Part model, mm, in its own coordinate system. Face numbers are marked on the shaded views. A direction names the side the tool comes from. Round coordinates to 2 decimals unless told otherwise and drop trailing zeros. Loops run counter-clockwise (first coordinate to the right, second up) from the corner with the lowest first, then second, coordinate; pieces in that order, holes last. Notation, with made-up numbers: M 28,-5 L 37,-5 A13 ccw 37,11 Z; hole C 21,73.25 d9. An arc over 180 degrees is marked long. Put each result on its own line as item: value. Start each with the question number.
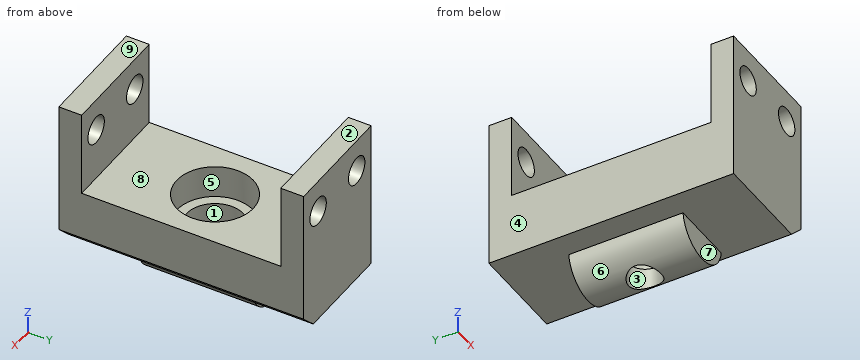
```python
from build123d import *

# Parameters (mm, degrees)
CYLINDER036_R          = 3.5
CYLINDER036_DEPTH      = 30
CYLINDER035_R          = 4.7
CYLINDER035_DEPTH      = 30
CYLINDER065_R          = 2
CYLINDER065_DEPTH      = 62
CYLINDER066_R          = 4
CYLINDER066_DEPTH      = 14
CYLINDER066_ROLL_ANGLE = 90
CYLINDER030_R          = 1.7
CYLINDER030_DEPTH      = 19
CYLINDER030_ROLL_ANGLE = 90
CYLINDER033_R          = 1.7
CYLINDER033_DEPTH      = 19
CYLINDER033_ROLL_ANGLE = 90
CYLINDER034_R          = 1.7
CYLINDER034_DEPTH      = 19
CYLINDER034_ROLL_ANGLE = 90
CYLINDER029_R          = 1.7
CYLINDER029_DEPTH      = 19
CYLINDER029_ROLL_ANGLE = 90
BOX001012_W            = 14
BOX001012_H            = 2.8
BOX001012_DEPTH        = 11
BOX001011_W            = 14
BOX001011_H            = 2.8
BOX001011_DEPTH        = 11
BOX001010_W            = 14
BOX001010_H            = 30
BOX001010_DEPTH        = 8
CHAMFER011_SIZE        = 2


with BuildPart() as cylinder036:
    # Cylinder036 → Cylinder036 (new body)
    with BuildSketch(Plane.XY.offset(-9)):
        Circle(CYLINDER036_R)
    extrude(amount=CYLINDER036_DEPTH)


with BuildPart() as bearing_nut:
    # Cylinder035 → Cylinder035 (new body)
    with BuildSketch(Plane.XY.offset(-4.5)):
        Circle(CYLINDER035_R)
    extrude(amount=CYLINDER035_DEPTH)

    # Fusion080: union Cylinder036
    add(cylinder036.part)


with BuildPart() as cylinder065:
    # Cylinder065 → Cylinder065 (new body)
    with BuildSketch(Plane.XY.offset(-59)):
        Circle(CYLINDER065_R)
    extrude(amount=CYLINDER065_DEPTH)


with BuildPart() as cut035:
    # Cylinder066 → Cylinder066 (new body)
    with BuildSketch(Plane.XY):
        Circle(CYLINDER066_R)
    extrude(amount=CYLINDER066_DEPTH)


with BuildPart() as cut035_1:
    # Cylinder066 roll: moved
    add(cut035.part.rotate(Axis((0, 0, 0), (1, 0, 0)), CYLINDER066_ROLL_ANGLE))


with BuildPart() as cut035_2:
    # Cylinder066 placement: moved
    add(cut035_1.part.moved(Location((0, 7, -8))))

    # Cut035: cut Cylinder065
    add(cylinder065.part, mode=Mode.SUBTRACT)


with BuildPart() as cylinder030:
    # Cylinder030 → Cylinder030 (new body)
    with BuildSketch(Plane.XY):
        Circle(CYLINDER030_R)
    extrude(amount=CYLINDER030_DEPTH)


with BuildPart() as cylinder030_1:
    # Cylinder030 roll: moved
    add(cylinder030.part.rotate(Axis((0, 0, 0), (1, 0, 0)), CYLINDER030_ROLL_ANGLE))


with BuildPart() as cylinder030_2:
    # Cylinder030 placement: moved
    add(cylinder030_1.part.moved(Location((4, 24, 6))))


with BuildPart() as cylinder033:
    # Cylinder033 → Cylinder033 (new body)
    with BuildSketch(Plane.XY):
        Circle(CYLINDER033_R)
    extrude(amount=CYLINDER033_DEPTH)


with BuildPart() as cylinder033_1:
    # Cylinder033 roll: moved
    add(cylinder033.part.rotate(Axis((0, 0, 0), (1, 0, 0)), CYLINDER033_ROLL_ANGLE))


with BuildPart() as cylinder033_2:
    # Cylinder033 placement: moved
    add(cylinder033_1.part.moved(Location((4, 24, 6))))


with BuildPart() as part_mirroring002:
    # Part__Mirroring002: instance of Cylinder033
    add(cylinder033_2.part.mirror(Plane(origin=(0, 0, 0), x_dir=(1, 0, 0), z_dir=(0, 1, 0))))


with BuildPart() as cylinder034:
    # Cylinder034 → Cylinder034 (new body)
    with BuildSketch(Plane.XY):
        Circle(CYLINDER034_R)
    extrude(amount=CYLINDER034_DEPTH)


with BuildPart() as cylinder034_1:
    # Cylinder034 roll: moved
    add(cylinder034.part.rotate(Axis((0, 0, 0), (1, 0, 0)), CYLINDER034_ROLL_ANGLE))


with BuildPart() as cylinder034_2:
    # Cylinder034 placement: moved
    add(cylinder034_1.part.moved(Location((-4, 24, 6))))


with BuildPart() as part_mirroring003:
    # Part__Mirroring003: instance of Cylinder034
    add(cylinder034_2.part.mirror(Plane(origin=(0, 0, 0), x_dir=(1, 0, 0), z_dir=(0, 1, 0))))


with BuildPart() as m3_clear_a:
    # Cylinder029 → Cylinder029 (new body)
    with BuildSketch(Plane.XY):
        Circle(CYLINDER029_R)
    extrude(amount=CYLINDER029_DEPTH)


with BuildPart() as m3_clear_a_1:
    # Cylinder029 roll: moved
    add(m3_clear_a.part.rotate(Axis((0, 0, 0), (1, 0, 0)), CYLINDER029_ROLL_ANGLE))


with BuildPart() as m3_clear_a_2:
    # Cylinder029 placement: moved
    add(m3_clear_a_1.part.moved(Location((-4, 24, 6))))

    # Fusion057: union Cylinder030, Part__Mirroring002, Part__Mirroring003
    add(cylinder030_2.part)
    add(part_mirroring002.part)
    add(part_mirroring003.part)


with BuildPart() as cube010:
    # Box001012 → Box001012 (new body)
    with BuildSketch(Plane(origin=(-7, 12.2, -1), x_dir=(1, 0, 0), z_dir=(0, 0, 1))):
        with Locations((7, 1.4)):
            Rectangle(BOX001012_W, BOX001012_H)
    extrude(amount=BOX001012_DEPTH)


with BuildPart() as cube009:
    # Box001011 → Box001011 (new body)
    with BuildSketch(Plane(origin=(-7, -15, -1), x_dir=(1, 0, 0), z_dir=(0, 0, 1))):
        with Locations((7, 1.4)):
            Rectangle(BOX001011_W, BOX001011_H)
    extrude(amount=BOX001011_DEPTH)


with BuildPart() as bearing_clamp:
    # Box001010 → Box001010 (new body)
    with BuildSketch(Plane(origin=(-7, -15, -8.5), x_dir=(1, 0, 0), z_dir=(0, 0, 1))):
        with Locations((7, 15)):
            Rectangle(BOX001010_W, BOX001010_H)
    extrude(amount=BOX001010_DEPTH)

    # Fusion055: union Cube010, Cube009
    add(cube010.part)
    add(cube009.part)

    # Cut006: cut M3-clear-a
    add(m3_clear_a_2.part, mode=Mode.SUBTRACT)

    # Fusion081: union Cut035
    add(cut035_2.part)

    # Cut036: cut bearing-nut
    add(bearing_nut.part, mode=Mode.SUBTRACT)

    # Chamfer011
    chamfer011_edges = [bearing_clamp.edges().sort_by_distance(p)[0] for p in [
        (7, 0, -8.5),
    ]]
    chamfer(chamfer011_edges, length=CHAMFER011_SIZE)


solid = bearing_clamp.part
```
1. Cut at B-B, the plane x = 0. Give the cut face in (y, z), and give its area (3 significant figures).
2. Wall check: L1, parallel to Z at x = 4, y = -12.75; L2, parallel to Y at x = -1, z = -0.25; L3, parallel to Y at x = 0, z = -11.2. Give the ranges that are in metal, low to high.
3. Cut at C-C, the plane y = -0.5. Give the cut face in (x, z), and give its area (3 significant figures).
4. Cut at A-A, the plane z = 1.5. Give the cut face in (x, y), and give its area (3 significant figures).
5. Mould opens along X. For the marked faces 1, 2, 3 and 4 say: released by +X, released by -X, zero draft, split by the parting line, or undercut.
6. Drop flat-ended pins along their axis: pin 1 (2.5 mm diameter, centred on x = -4, z = 6, fed in from +Y); pin 2 (5 mm diameter, centred on x = 1, y = -5.5, fed in from +Z); pin 3 (3 mm diameter, centred on x = -1, z = -11, fed in from +Y); pin 4 (6 mm diameter, centred on x = -3.5, y = 7, fed in from -Z). Give the stop position or say it passes through.
7. Cut at D-D, the plane z = 6. Give the cut face in (x, y), and give its area (3 significant figures).
8. Which spindle directions (+Z, -Z, +X, -X, +Y, -Y) get a long thin tool onto all of the face, cutting with end or side? Do the marked faces 5, 6, 7, 8 and 9. Say none if no direction does.
Results list:
1. outline: M -15,-8.5 L -7,-8.5 L -7,-12 L -2,-12 L -2,-9 L -3.5,-9 L -3.5,-4.5 L -4.7,-4.5 L -4.7,-0.5 L -12.2,-0.5 L -12.2,10 L -15,10 Z; M 2,-12 L 7,-12 L 7,-8.5 L 15,-8.5 L 15,10 L 12.2,10 L 12.2,-0.5 L 4.7,-0.5 L 4.7,-4.5 L 3.5,-4.5 L 3.5,-9 L 2,-9 Z
1. area: 267 mm^2
2. L1: z = -8.5 to 4.3, 7.7 to 10
2. L2: y = -15 to -12.2, 12.2 to 15
2. L3: y = -7 to -2, 2 to 7
3. outline: M -7,-8.5 L -3.97,-8.5 A4 ccw -1.94,-11.5 L -1.94,-9 L -3.46,-9 L -3.46,-4.5 L -4.67,-4.5 L -4.67,-0.5 L -7,-0.5 Z; M 1.94,-11.5 A4 ccw 3.97,-8.5 L 5,-8.5 L 7,-6.5 L 7,-0.5 L 4.67,-0.5 L 4.67,-4.5 L 3.46,-4.5 L 3.46,-9 L 1.94,-9 Z
3. area: 51.6 mm^2
4. outline: M -7,-15 L 7,-15 L 7,-12.2 L -7,-12.2 Z; M -7,12.2 L 7,12.2 L 7,15 L -7,15 Z
4. area: 78.4 mm^2
5. face 1: undercut
5. face 2: zero draft
5. face 3: undercut
5. face 4: released by -X
6. pin 1: passes through
6. pin 2: stops at z = -0.5
6. pin 3: stops at y = 7
6. pin 4: stops at z = -11.97
7. outline: M -7,-15 L -5.7,-15 L -5.7,-12.2 L -7,-12.2 Z; M -7,12.2 L -5.7,12.2 L -5.7,15 L -7,15 Z; M -2.3,-15 L 2.3,-15 L 2.3,-12.2 L -2.3,-12.2 Z; M -2.3,12.2 L 2.3,12.2 L 2.3,15 L -2.3,15 Z; M 5.7,-15 L 7,-15 L 7,-12.2 L 5.7,-12.2 Z; M 5.7,12.2 L 7,12.2 L 7,15 L 5.7,15 Z
7. area: 40.3 mm^2
8. face 5: +Z
8. face 6: -Z, +Y, -Y
8. face 7: -Z, +X, -X, -Y
8. face 8: +Z, +X, -X
8. face 9: +Z, +X, -X, +Y, -Y
